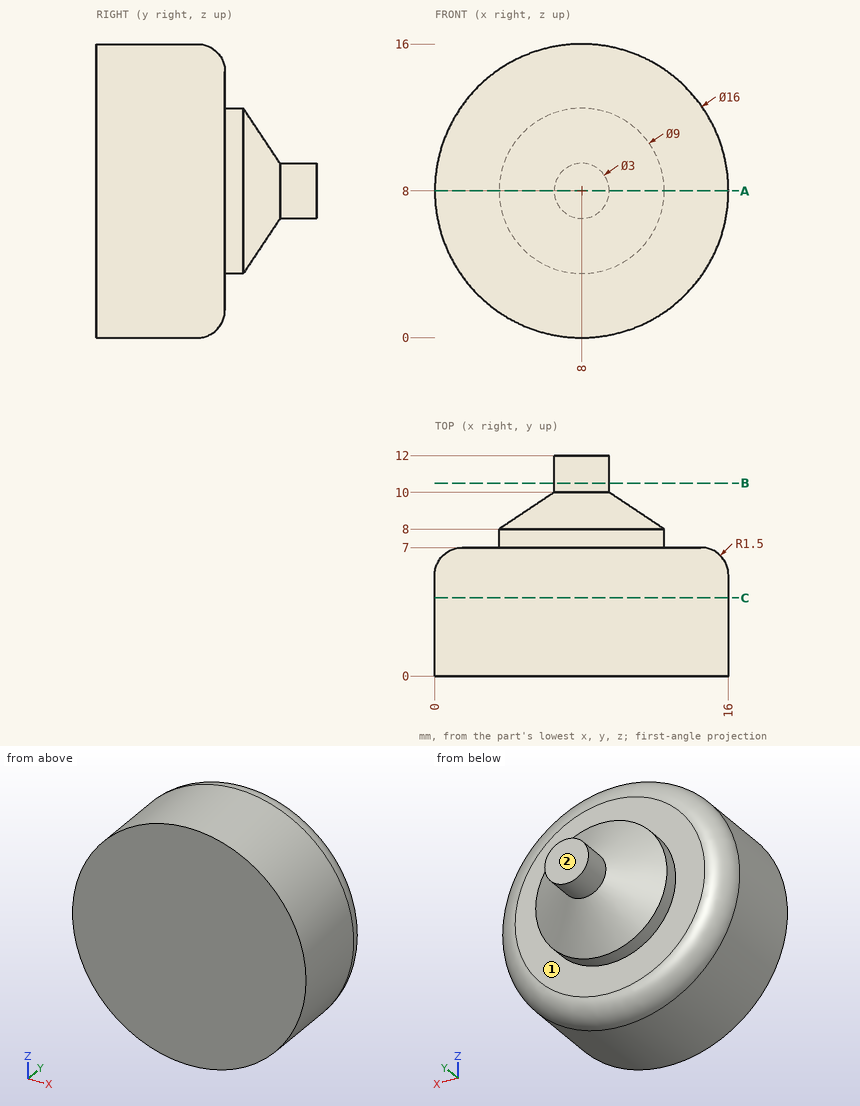
Answer from the drawing. Dimensions are ordinates in mm from the lowest x, y and z of the part. A direction names the side the tool comes from. Round coordinates to 2 decimals unless told otherwise and drop trailing zeros. Loops run counter-clockwise (first coordinate to the right, second up) from the corner with the lowest first, then second, coordinate; pieces in that order, holes last. Notation, with made-up numbers: M -22,-19 L 13,-19 A23 ccw 13,4 Z; hole C -22,55.25 d6. An arc over 180 degrees is marked long. One line per question, with ' | ' between items. Start each with the question number.
(1) Flat-ended cylindrical pins translate along their axes: pin 1 Ø1 at (y, z) = (8, 7) entering from +X; pin 2 Ø6 at (x, y) = (2, 3.5) entering from -Z; pin 3 Ø6 at (y, z) = (9.5, 5) entering from -X. Find the tip coordinate at first contact, or state that the pin passes through.
(2) A cutting plane is placed at B-B on y = 10.5. Write down the section's boundary in (x, z), plus the area to 3 significant figures.
(3) A cutting plane is placed at C-C on y = 4.25. Write down the section's boundary in (x, z).
(4) A tool of negligible diameter and unlimited length cuts with its end or side. For the marked faces 1 and 2, from which of +Z, -Z, +X, -X, +Y, -Y can it reach the whole face along a straight path? Write none if from no direction.
(5) Find the intervals of material crossed by line 1 (Y direction, x = 14, z = 5.5); line 2 (Y direction, x = 3.5, z = 2.5); line 3 (Z direction, x = 7.25, y = 2.5), in increasing order.
(6) A cutting plane is placed at A-A on z = 8. Write down the section's boundary in (x, y), plus the area to 3 significant figures.
Geometry check:
1) pin 1: stops at x = 12.47 | pin 2: stops at z = 0.58 | pin 3: stops at x = 0.82
2) outline: C 8,8 d3 | area: 7.07 mm²
3) outline: C 8,8 d16
4) face 1: +Y | face 2: +Z, -Z, +X, -X, +Y
5) line 1: y = 0 to 7 | line 2: y = 0 to 6.87 | line 3: z = 0.04 to 15.96
6) outline: M 0,0 L 16,0 L 16,5.5 A1.5 ccw 14.5,7 L 12.5,7 L 12.5,8 L 9.5,10 L 9.5,12 L 6.5,12 L 6.5,10 L 3.5,8 L 3.5,7 L 1.5,7 A1.5 ccw 0,5.5 Z | area: 138 mm²
